Solid Edge part; units mm, degrees
sketch "Sketch1" plane through (0, 0, 0) normal (0, -1, 0) x (1, 0, 0)
  line L0 (30.8823, 2) -> (-19.5736, 52.4558)
  line L1 (-37, 52.4558) -> (-19.5736, 52.4558)
  line L2 (-37, 52.4558) -> (-37, 27.4558)
  line L3 (-37, 27.4558) -> (-11.5442, 2)
  line L4 (-11.5442, 2) -> (30.8823, 2)
extrude "Protrusion1" add sketch "Sketch1" along normal mid plane 3
sketch "Sketch2" plane through (0, 0, 0) normal (0, -1, 0) x (1, 0, 0)
  line L0 (-22, 17) -> (-37, 17)
  line L1 (-37, 17) -> (-37, 2)
  line L2 (-37, 2) -> (-22, 2)
  line L3 (-22, 2) -> (-22, 17)
extrude "Cutout1" cut sketch "Sketch2" against normal up to next and the other way up to next
Verification items for the finished model (mm, model axes). A direction names the side the tool comes from. Coordinates: 2 decimals unless noted, no trailing zeros. Order: outer loops, then holes, each group sorted by start corner. A loop starts at its lowest first (then second) coordinate and runs counter-clockwise, first axis right, second up. Notation, with made-up numbers: M -21.5,8 L -4.5,8 A15 cw -4.5,18 Z; hole C -24.75,-20 d7. An arc over 180 degrees is marked long. One line per item, written item: value. Start each with the question number.
Item 1: Sectioned sample at B-B on x = -31. Record the cut outline in (y, z), then the cut area to 3 significant figures.
Item 2: Depth check by flat-ended pin: P1, Ø0.9, axis at y = -0.5, z = 16, coming from the -X side; P2, Ø1.5, axis at x = -24.5, y = 0, coming from the -Z side. Enter the tip coordinate at first touch or a pass-through.
Item 3: Access from +Z, -Z, +X, -X, +Y, -Y to the whole of each face (thin tool, end or side, straight path). Record for faces 1 (the flat face through (-24, 0, 17)), 2 (the flat face through (6.01, 0.02, 26.87)).
Item 4: Sectioned sample at C-C on z = 30. Record the cut outline in (x, y).
Item 5: Thickness scan on probe 1 along Z at (x, y) = (23, 0.3); probe 2 along X at (y, z) = (-1.3, 48); probe 3 along Z at (x, y) = (-28, 0.3). Record the ranges inside material, lowest first.
Item 6: Sectioned sample at A-A on y = 0.45. Record the cut outline in (x, z), then the cut area to 3 significant figures.
Calculated:
1. outline: M -1.5,21.46 L 1.5,21.46 L 1.5,52.46 L -1.5,52.46 Z
1. area: 93.0 mm^2
2. P1: x = -22
2. P2: z = 17
3. face 1: -Z, -X, +Y, -Y
3. face 2: +Z, +X, +Y, -Y
4. outline: M -37,-1.5 L 2.88,-1.5 L 2.88,1.5 L -37,1.5 Z
5. probe 1: 2 to 9.88
5. probe 2: -37 to -15.12
5. probe 3: 18.46 to 52.46
6. outline: M -37,27.46 L -26.54,17 L -22,17 L -22,12.46 L -11.54,2 L 30.88,2 L -19.57,52.46 L -37,52.46 Z
6. area: 1,820 mm^2
